Work out the finished part from the listing and answer in its coordinate system (mm). A direction names the side the tool comes from. Give positions to 0.01 mm unless a question says otherwise; leave off trailing zeros. Loops run counter-clockwise (first coordinate to the right, second up) from the corner with the lowest first, then second, coordinate; pieces in that order, holes last. Notation, with made-up numbers: (16, 11) - (70, 11) arc R12 cw to (70, 26) - close; hole circle Ø8 at (10.25, 32). An arc over 180 degrees is marked (long way). One line per question, with ' | ' between items. Start each with the question number.
1. Section C-C (z = 7.5) is taken. Give the number of separate pieces and of enclosed holes in the cut face, plus the area to 3 significant figures.
2. For a pull along Y with two mould halves and no side action, classify faces 5 (the face through (28.81, -28.2, 33.52)), 6 (the face through (-2, 45, 38)), 7 (the face through (-2, 35, 0)) as released by +Y, released by -Y, zero draft, split by the parting line, or undercut.
3. Section B-B (z = 53) is taken. Determine the outline of the cut face in (x, y).
4. Each of these flat-tipped pins is pushed along its axis until it touches: pin 1 (8 mm diameter, centred on x = 91.5, y = 30, fed in from -Z); pin 2 (6 mm diameter, centred on y = 16, z = 57, fed in from -X); pin 3 (5.5 mm diameter, centred on x = -95.5, y = 13, fed in from -Z); pin 4 (2.5 mm diameter, centred on x = -92.5, y = -29.5, fed in from -Z). Where does it stop, or does it pass through?
5. Which of the six approach directions +Z, -Z, +X, -X, +Y, -Y give full straight-line access (tool end or side, diameter ignored) to faces 1 (the face through (-28.81, 28.2, 33.52)), 2 (the face through (0, 0, 2.5)), 3 (the face through (-73.594, -16.691, 76.578)), 4 (the face through (99.896, 11.831, 13.839))?
6. Find the intervals of material crossed by line 1 (X direction, y = -30, z = 15); line 2 (Y direction, x = 96, z = 15); line 3 (Y direction, x = -96.5, z = 13.25), in increasing order.
7. Section D-D (z = 65) is taken. Determine the outline of the cut face in (x, y), plus the area to 3 significant figures.
8. Section A-A (x = -39.5) is taken. Determine the outline of the cut face in (y, z), plus the area to 3 significant figures.
from build123d import *

# Parameters (mm, degrees)
F0_W      = 220
F0_H      = 90
F1_DEPTH  = 80
F3_DEPTH  = 80.001
F4_R      = 12
F6_DEPTH  = 90
F8_DEPTH  = 220.001
F9_R      = 2.465
F10_DEPTH = 23.18
F11_R     = 2.465
F12_DEPTH = 23.5
F13_R     = 2.43
F14_DEPTH = 23
F13_R_2   = 3.56
F15_DEPTH = 25.5


# Not quite as in the source:
# - a feature names something its author has since deleted; it is built from what else it names


with BuildPart() as f1:
    # F0 (on Top) → F1 (new body)
    with BuildSketch(Plane.XY):
        Rectangle(F0_W, F0_H)
    extrude(amount=F1_DEPTH)

    # F2 (on face) → F3 (cut, through all)
    with BuildSketch(Plane(origin=(0, 0, 0), x_dir=(1, 0, 0), z_dir=(0, 0, -1))):
        with BuildLine():
            ThreePointArc((-13.8230854638, -5), (-12.8240812387, -2.588190451), (-12.4833395016, 0))
            Line((-12.4833395016, 0), (-45, 0))
            Line((-45, 0), (-45, 29.5))
            Line((-45, 29.5), (-56.2583302492, 29.5))
            ThreePointArc((-56.2583302492, 29.5), (-61.2583302492, 28.1602540378), (-64.918584287, 24.5))
            Line((-64.918584287, 24.5), (-76.1769145362, 5))
            ThreePointArc((-76.1769145362, 5), (-77.5166604984, 0), (-76.1769145362, -5))
            Line((-76.1769145362, -5), (-64.918584287, -24.5))
            ThreePointArc((-64.918584287, -24.5), (-61.2583302492, -28.1602540378), (-56.2583302492, -29.5))
            Line((-56.2583302492, -29.5), (-33.7416697508, -29.5))
            ThreePointArc((-33.7416697508, -29.5), (-28.7416697508, -28.1602540378), (-25.081415713, -24.5))
            Line((-25.081415713, -24.5), (-13.8230854638, -5))
        make_face()
        with BuildLine():
            Line((-45, 0), (-12.4833395016, 0))
            ThreePointArc((-12.4833395016, 0), (-12.8240812387, 2.588190451), (-13.8230854638, 5))
            Line((-13.8230854638, 5), (-25.081415713, 24.5))
            ThreePointArc((-25.081415713, 24.5), (-28.7416697508, 28.1602540378), (-33.7416697508, 29.5))
            Line((-33.7416697508, 29.5), (-45, 29.5))
            Line((-45, 29.5), (-45, 0))
        make_face()
        with BuildLine():
            ThreePointArc((13.8230854638, 5), (12.8240812387, 2.588190451), (12.4833395016, 0))
            Line((12.4833395016, 0), (45, 0))
            Line((45, 0), (45, 29.5))
            Line((45, 29.5), (33.7416697508, 29.5))
            ThreePointArc((33.7416697508, 29.5), (28.7416697508, 28.1602540378), (25.081415713, 24.5))
            Line((25.081415713, 24.5), (13.8230854638, 5))
        make_face()
        with BuildLine():
            Line((45, 0), (12.4833395016, 0))
            ThreePointArc((12.4833395016, 0), (12.8240812387, -2.588190451), (13.8230854638, -5))
            Line((13.8230854638, -5), (25.081415713, -24.5))
            ThreePointArc((25.081415713, -24.5), (28.7416697508, -28.1602540378), (33.7416697508, -29.5))
            Line((33.7416697508, -29.5), (56.2583302492, -29.5))
            ThreePointArc((56.2583302492, -29.5), (61.2583302492, -28.1602540378), (64.918584287, -24.5))
            Line((64.918584287, -24.5), (76.1769145362, -5))
            ThreePointArc((76.1769145362, -5), (77.5166604984, 0), (76.1769145362, 5))
            Line((76.1769145362, 5), (64.918584287, 24.5))
            ThreePointArc((64.918584287, 24.5), (61.2583302492, 28.1602540378), (56.2583302492, 29.5))
            Line((56.2583302492, 29.5), (45, 29.5))
            Line((45, 29.5), (45, 0))
        make_face()
    extrude(amount=-F3_DEPTH, mode=Mode.SUBTRACT)

    # F4
    f4_edges = [f1.edges().sort_by_distance(p)[0] for p in [
        (-45, 29.5, 80),
        (45, 29.5, 80),
    ]]
    fillet(f4_edges, radius=F4_R)

    # F5 (on face) → F6 (cut)
    with BuildSketch(Plane.XZ.offset(45)):
        Polygon((-110, 80), (-110, 50), (-96.0107702554, 80), align=None)
        Polygon((110, 80), (93.621339458, 80), (110, 35), align=None)
    extrude(amount=-F6_DEPTH, mode=Mode.SUBTRACT)

    # F7 (on face) → F8 (cut, through all)
    with BuildSketch(Plane(origin=(-110, 0, 0), x_dir=(0, -1, 0), z_dir=(-1, 0, 0))):
        Polygon((-23.5, 80), (-45, 80), (-45, 76.2089699148), align=None)
        Polygon((23.5, 80), (45, 76.2089699148), (45, 78.1686380506), (45, 80), align=None)
        Polygon((-24, 0), (0, 0), (24, 0), (24, 2.5), (-24, 2.5), align=None)
    extrude(amount=-F8_DEPTH, mode=Mode.SUBTRACT)

    # F9 (on face) → F10 (cut)
    with BuildSketch(Plane(origin=(-110, 0, 0), x_dir=(0, -1, 0), z_dir=(-1, 0, 0))):
        with Locations((0, 47)):
            Circle(F9_R)
    extrude(amount=-F10_DEPTH, mode=Mode.SUBTRACT)

    # F11 (on face) → F12 (cut)
    with BuildSketch(Plane.XZ.offset(45)):
        with Locations((0, 59.465)):
            Circle(F11_R)
    extrude(amount=-F12_DEPTH, mode=Mode.SUBTRACT)

    # F13 (on face) → F14 (cut)
    with BuildSketch(Plane(origin=(0, 0, 0), x_dir=(1, 0, 0), z_dir=(0, 0, -1))):
        with Locations((-91.5, 30)):
            Circle(F13_R)
        with Locations((91.5, 30)):
            Circle(F13_R)
        with Locations((91.5, -30)):
            Circle(F13_R)
        with Locations((-91.5, -30)):
            Circle(F13_R)
    extrude(amount=-F14_DEPTH, mode=Mode.SUBTRACT)

    # F13 (on face) → F15 (cut)
    with BuildSketch(Plane(origin=(0, 0, 0), x_dir=(1, 0, 0), z_dir=(0, 0, -1))):
        with Locations((-96.5, 12.9)):
            Circle(F13_R_2)
        with Locations((-96.5, -12.9)):
            Circle(F13_R_2)
        with Locations((96.5, -12.9)):
            Circle(F13_R_2)
        with Locations((96.5, 12.9)):
            Circle(F13_R_2)
    extrude(amount=-F15_DEPTH, mode=Mode.SUBTRACT)


solid = f1.part
Conclusion:
1) separate pieces: 1 | enclosed holes: 10 | area: 13,600 mm²
2) face 5: undercut | face 6: released by +Y | face 7: zero draft
3) outline: (-108.6, -45) - (103.45, -45) - (103.45, 45) - (-108.6, 45) - close; hole (-76.18, -5) - (-64.92, -24.5) arc R10 ccw to (-56.26, -29.5) - (-33.74, -29.5) arc R10 ccw to (-25.08, -24.5) - (-13.82, -5) arc R10 ccw to (-13.82, 5) - (-25.08, 24.5) arc R10 ccw to (-33.74, 29.5) - (-56.26, 29.5) arc R10 ccw to (-64.92, 24.5) - (-76.18, 5) arc R10 ccw to start; hole (13.82, -5) - (25.08, -24.5) arc R10 ccw to (33.74, -29.5) - (56.26, -29.5) arc R10 ccw to (64.92, -24.5) - (76.18, -5) arc R10 ccw to (76.18, 5) - (64.92, 24.5) arc R10 ccw to (56.26, 29.5) - (33.74, 29.5) arc R10 ccw to (25.08, 24.5) - (13.82, 5) arc R10 ccw to start
4) pin 1: z = 0 | pin 2: x = -108.13 | pin 3: z = 2.5 | pin 4: z = 23
5) face 1: +Z, -Z | face 2: -Z, +X, -X | face 3: +Z | face 4: -Z
6) line 1: -110 to -93.93, -89.07 to 89.07, 93.93 to 110 | line 2: -45 to -16.42, -9.38 to 9.38, 16.42 to 45 | line 3: -45 to -16.46, -9.34 to 9.34, 16.46 to 45
7) outline: (-103.01, -45) - (99.08, -45) - (99.08, 45) - (-103.01, 45) - close; hole (-76.18, -5) - (-64.92, -24.5) arc R10 ccw to (-56.26, -29.5) - (-33.74, -29.5) arc R10 ccw to (-25.08, -24.5) - (-13.82, -5) arc R10 ccw to (-13.82, 5) - (-25.08, 24.5) arc R10 ccw to (-33.74, 29.5) - (-56.26, 29.5) arc R10 ccw to (-64.92, 24.5) - (-76.18, 5) arc R10 ccw to start; hole (13.82, -5) - (25.08, -24.5) arc R10 ccw to (33.74, -29.5) - (56.26, -29.5) arc R10 ccw to (64.92, -24.5) - (76.18, -5) arc R10 ccw to (76.18, 5) - (64.92, 24.5) arc R10 ccw to (56.26, 29.5) - (33.74, 29.5) arc R10 ccw to (25.08, 24.5) - (13.82, 5) arc R10 ccw to start | area: 12,200 mm²
8) outline: (-45, 0) - (-29.5, 0) - (-29.5, 68) arc R12 ccw to (-34.86, 78) - (-45, 76.21) - close; (29.5, 0) - (45, 0) - (45, 76.21) - (34.86, 78) arc R12 ccw to (29.5, 68) - close | area: 2,370 mm²
